```python
from build123d import *

# Parameters (mm, degrees)
PAD007_DEPTH    = 15
FILLET004_R     = 5
SKETCH016_R     = 3.2
POCKET007_DEPTH = 9.001
SKETCH017_R     = 6.5
POCKET008_DEPTH = 231.001


with BuildPart() as part:
    # Sketch015 → Pad007 (new body, symmetric)
    with BuildSketch(Plane.XY):
        with BuildLine():
            Line((231, 76.944483), (231, 80.944483))
            Line((231, 95.944483), (231, 80.944483))
            Line((227, 95.944483), (231, 95.944483))
            Line((227, 80.944483), (227, 95.944483))
            Line((227, 80.944483), (-4, 80.944483))
            Line((-4, 80.944483), (-4, -79.894546))
            Line((-4, -79.894546), (0, -79.894546))
            ThreePointArc((231, 76.944483), (101.370956, 19.334898), (0, -79.894546))
        make_face()
        with BuildLine():
            Line((0, -73.055517), (0, 0))
            ThreePointArc((0, 0), (20.003059, 0.422481), (39.624191, 4.335541))
            Line((39.624191, 4.335541), (53.376827, -13.501329))
            ThreePointArc((53.376827, -13.501329), (25.211158, -41.954399), (0, -73.055517))
        make_face(mode=Mode.SUBTRACT)
        with BuildLine():
            Line((2, 76.944483), (111.264747, 76.944483))
            ThreePointArc((2, 3.888966), (68.743581, 22.302719), (111.264747, 76.944483))
            Line((2, 3.888966), (2, 76.944483))
        make_face(mode=Mode.SUBTRACT)
        with BuildLine():
            ThreePointArc((215.369261, 76.944483), (159.431544, 56.441008), (107.117433, 27.933914))
            Line((96.234655, 42.048639), (107.117433, 27.933914))
            ThreePointArc((96.234655, 42.048639), (107.404352, 58.647999), (115.5, 76.944483))
            Line((115.5, 76.944483), (215.369261, 76.944483))
        make_face(mode=Mode.SUBTRACT)
        with BuildLine():
            Line((93.602426, 38.911672), (103.756041, 25.742655))
            ThreePointArc((103.756041, 25.742655), (79.375609, 8.346637), (56.350936, -10.807771))
            Line((43.69293, 5.609386), (56.350936, -10.807771))
            ThreePointArc((43.69293, 5.609386), (70.877923, 18.918104), (93.602426, 38.911672))
        make_face(mode=Mode.SUBTRACT)
    extrude(amount=PAD007_DEPTH, both=True)

    # Fillet004
    fillet004_edges = [part.edges().sort_by_distance(p)[0] for p in [
        (2, 76.944483, 0),
        (111.264747, 76.944483, 0),
        (115.5, 76.944483, 0),
        (2, 3.888966, 0),
        (0, 0, 0),
        (43.69293, 5.609386, 0),
        (39.624191, 4.335541, 0),
        (96.234655, 42.048639, 0),
        (93.602426, 38.911672, 0),
        (215.369261, 76.944483, 0),
        (0, -73.055517, 0),
        (53.376827, -13.501329, 0),
        (56.350936, -10.807771, 0),
        (103.756041, 25.742655, 0),
        (107.117433, 27.933914, 0),
    ]]
    fillet(fillet004_edges, radius=FILLET004_R)

    # Sketch016 → Pocket007 (cut, through all)
    with BuildSketch(Plane.YZ.offset(5)):
        with Locations((-60, 0)):
            Circle(SKETCH016_R)
        with Locations((60, 0)):
            Circle(SKETCH016_R)
    extrude(amount=-POCKET007_DEPTH, mode=Mode.SUBTRACT)

    # Sketch017 → Pocket008 (cut, through all)
    with BuildSketch(Plane.YZ):
        with Locations((-60, 0)):
            Circle(SKETCH017_R)
    extrude(amount=POCKET008_DEPTH, mode=Mode.SUBTRACT)


solid = part.part
```
The listing builds one solid part. Answer for the finished solid, in the listing's coordinates (mm). A direction names the side the tool comes from. Give positions to 0.01 mm unless a question says otherwise; leave off trailing zeros. Order: outer loops, then holes, each group sorted by start corner. A loop starts at its lowest first (then second) coordinate and runs counter-clockwise, first axis right, second up.
1) Find section A-A on x = 174.5. Write down the section's boundary in (y, z).
Reported:
outline: (58.58, -15) - (62.9, -15) - (62.9, 15) - (58.58, 15) - close; (76.94, -15) - (80.94, -15) - (80.94, 15) - (76.94, 15) - close
2) Determine the mould class of faces 1 (the face through (9.4, -66.3, 1.6)), 2 (the face through (116.14, 76.03, -0.21)) for opening direction Z: pulls with the +Z half, pulls with the -Z half, needs draft (parallel to the pull), parting line crosses it, or undercut.
Reported:
face 1: undercut
face 2: needs draft
3) Find section B-B on x = 93.5. Write down the section's boundary in (y, z).
Reported:
outline: (13.85, -15) - (18.76, -15) - (18.76, 15) - (13.85, 15) - close; (36.15, -15) - (45.03, -15) - (45.03, 15) - (36.15, 15) - close; (76.94, -15) - (80.94, -15) - (80.94, 15) - (76.94, 15) - close
4) Consider line 1 along Z through (x, y) = (-2, 60); line 2 along Y through (x, z) = (6, 0); line 3 along Y through (x, z) = (9.25, 0). Determine where each line is inside the solid, lowest interval first.
Reported:
line 1: z = -15 to -3.2, 3.2 to 15
line 2: y = -71.67 to -66.5, -0.24 to 3.85, 76.84 to 80.94
line 3: y = -67.4 to -66.5, -0.24 to 3.76, 76.94 to 80.94
5) Given P1, Ø6, axis at y = -28, z = 6, coming from the +X side; P2, Ø6, axis at y = 60, z = 0, coming from the -X side; P3, Ø2, axis at x = 83, z = 0, coming from the +Y side, each flat-ended and moving along its own axis, determine where each tip first touches the part or whether it passes through.
Reported:
P1: stops at x = 47.02
P2: stops at x = 101.84
P3: stops at y = 80.94
6) For faces 3 (the face through (71, 19, 0)), 4 (the face through (-2, -63.2, 0.1)), determine the directions among +Z, -Z, +X, -X, +Y, -Y from which every point of the face is accessible in a straight line to the end or side of a thin tool.
Reported:
face 3: +Z, -Z
face 4: +X, -X
7) Find section D-D on y = 60. Write down the section's boundary in (x, z).
Reported:
outline: (-4, -15) - (2, -15) - (2, -3.2) - (-4, -3.2) - close; (-4, 3.2) - (2, 3.2) - (2, 15) - (-4, 15) - close; (103.58, -15) - (108.14, -15) - (108.14, 15) - (103.58, 15) - close; (167.53, -15) - (178.02, -15) - (178.02, 15) - (167.53, 15) - close
8) Find section C-C on z = 0. Give the number of separate pieces and of enclosed holes in the cut face, then the cut area to 3 significant figures.
Reported:
separate pieces: 2
enclosed holes: 2
area: 3,690 mm2
